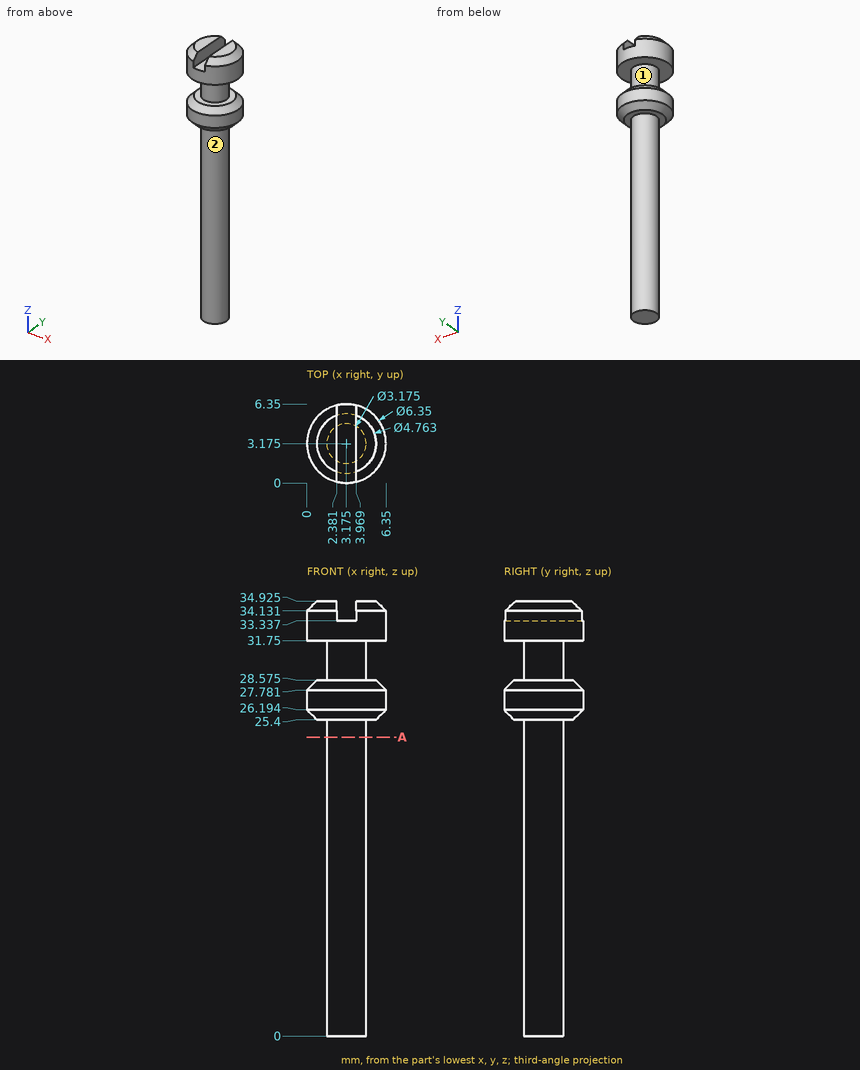
Could you check a few things on this drawing? It's one solid part, dimensions in mm from its lowest x, y, z. Give positions to 0.01 mm unless a question says otherwise; leave off trailing zeros. Write each loop counter-clockwise with the first axis right and the second up, starting at its lowest first coordinate (ties: lowest second). Pieces come first, ordered by that corner, then holes.
(1) Imagine slicing it at A-A, the plane z = 24. Write out the boundary of the cut face in (x, y) (1 decimal).
Output values:
outline: circle Ø3.2 at (3.2, 3.2)
(2) Thinking about a two-plate mould opening in Z: for the marked faces 1 and 2, which applies, pulls with the +Z half, pulls with the -Z half, needs draft (parallel to the pull), parting line crosses it, or undercut?
Output values:
face 1: undercut
face 2: needs draft
(3) Will these pins go through, and if not, where does the flat tip stop? pin 1 (1.4 mm diameter, centred on x = 4, y = 2.5, fed in from -Z); pin 2 (0.8 mm diameter, centred on x = 3.5, y = 3, fed in from +Z); pin 3 (1 mm diameter, centred on x = 2, z = 22.5, fed in from -Y); pin 4 (1.7 mm diameter, centred on y = 4.5, z = 34, fed in from +X) (1 decimal).
Output values:
pin 1: stops at z = 0
pin 2: stops at z = 33.34
pin 3: stops at y = 1.74
pin 4: stops at x = 6.3
(4) If I drill on L1, parallel to Y at x = 1.75, z = 21 (1 decimal); L2, parallel to Y at x = 6, z = 33.5 (1 decimal), over which ranges is the centre line in solid material (lowest first)?
Output values:
L1: y = 2.5 to 3.9
L2: y = 1.7 to 4.6
